The listing builds one solid part. Answer for the finished solid, in the listing's coordinates (mm). A direction names the side the tool comes from. Round coordinates to 2 decimals unless told otherwise and drop trailing zeros. Write each loop counter-clockwise with the first axis right and the second up, starting at its lowest first coordinate (ties: lowest second). Pieces come first, ordered by that corner, then holes.
Item 1: Find section B-B on z = 24.5. Give the vertices of the cut face in (x, y), then the cut area to 3 significant figures.
Item 2: Find section D-D on y = -7.75. Give the vertices of the cut face in (x, z).
Item 3: Find section C-C on y = 2.5. Give the vertices of the cut face in (x, z).
Item 4: Each of these flat-tipped pins is pushed along its axis until it touches: pin 1 (4 mm diameter, centred on y = -6, z = 25, fed in from -X); pin 2 (6 mm diameter, centred on y = -0.5, z = 8, fed in from -X); pin 3 (6 mm diameter, centred on y = 7.5, z = 6, fed in from +X); pin 4 (2 mm diameter, centred on x = 4, z = 9, fed in from -Y). Where does it stop, or does it pass through?
Item 5: For a pull along Y with two mould halves and no side action, classify faces 1 (the face through (0, 0, 0)), 2 (the face through (0.1, 9.8, 2.2)), 3 (the face through (9.54, 3, 14.79)) as +Y half, -Y half, draft (parallel to the pull), parting line (faces both ways), or undercut.
Item 6: Find section A-A on y = -4.25. Give the vertices of the cut face in (x, z), then the cut area to 3 significant figures.
Item 7: A tool of negligible diameter and unlimited length cuts with its end or side. For faces 4 (the face through (-0.65, -2.93, 16.68)), 5 (the face through (-2.42, -2.36, 4.74)), 6 (the face through (2.1, 2.4, 30)), from which of +Z, -Z, +X, -X, +Y, -Y can it reach the whole face along a straight path? Write none if from no direction.
Item 8: Find the intervals of material crossed by probe 1 along Z at (x, y) = (-3, -6); probe 2 along Y at (x, z) = (0, 20); probe 3 along Z at (x, y) = (-0.75, -1.25), in increasing order.
```python
from build123d import *

# Parameters (mm, degrees)
F0_R          = 10
F0_R_2        = 9.8
F0_R_3        = 3
F2_DEPTH      = 2
F3_DEPTH      = 30
F4_DEPTH      = 25
F4_DEPTH_BACK = 25
F5_DEPTH      = 2.5


with BuildPart() as f2:
    # F0 (on Top) → F2 (new body)
    with BuildSketch(Plane.XY):
        Circle(F0_R)
        Circle(F0_R_2, mode=Mode.SUBTRACT)
        Circle(F0_R_2)
        Circle(F0_R_3, mode=Mode.SUBTRACT)
        Circle(F0_R_3)
    extrude(amount=F2_DEPTH)

    # F0 (on Top) → F3 (join)
    with BuildSketch(Plane.XY):
        Circle(F0_R)
        Circle(F0_R_2, mode=Mode.SUBTRACT)
        Circle(F0_R_2)
        Circle(F0_R_3, mode=Mode.SUBTRACT)
    extrude(amount=F3_DEPTH)

    # F1 (on Front) → F4 (cut, two sides)
    with BuildSketch(Plane.XZ) as f4_sk:
        Polygon((-4, 2), (0, 2), (4, 2), (0, 8.9282032303), align=None)
    extrude(amount=F4_DEPTH, mode=Mode.SUBTRACT)
    extrude(f4_sk.sketch, amount=-F4_DEPTH_BACK, mode=Mode.SUBTRACT)

    # F0 (on Top) → F5 (join)
    with BuildSketch(Plane.XY):
        Circle(F0_R)
        Circle(F0_R_2, mode=Mode.SUBTRACT)
    extrude(amount=F5_DEPTH)


solid = f2.part
```
Check values:
1. outline: circle Ø20 at (0, 0); hole circle Ø6 at (0, 0)
1. area: 286 mm2
2. outline: (-6.32, 0) - (6.32, 0) - (6.32, 30) - (-6.32, 30) - close; hole (-4, 2) - (4, 2) - (0, 8.93) - close
3. outline: (-9.68, 0) - (9.68, 0) - (9.68, 30) - (1.66, 30) - (1.66, 6.06) - (4, 2) - (-4, 2) - (-1.66, 6.06) - (-1.66, 30) - (-9.68, 30) - close
4. pin 1: stops at x = -9.17
4. pin 2: stops at x = -10
4. pin 3: stops at x = 8.93
4. pin 4: stops at y = -9.54
5. face 1: draft
5. face 2: undercut
5. face 3: parting line
6. outline: (-9.05, 0) - (9.05, 0) - (9.05, 30) - (-9.05, 30) - close; hole (-4, 2) - (4, 2) - (0, 8.93) - close
6. area: 515 mm2
7. face 4: +Z
7. face 5: none
7. face 6: +Z, +X, -X, +Y, -Y
8. probe 1: z = 0 to 2, 3.73 to 30
8. probe 2: y = -10 to -3, 3 to 10
8. probe 3: z = 0 to 2
